from build123d import *

# Parameters (mm, degrees)
F1_DEPTH  = 3
F3_DEPTH  = 25
F4_R      = 5
F5_R      = 11.15
F5_R_2    = 2.65
F6_DEPTH  = 25
F7_W      = 78
F7_H      = 55.5
F7_R      = 2
F8_DEPTH  = 25
F9_R      = 8.15
F10_DEPTH = 25
F12_W     = 307.7535755343
F12_H     = 117.255145081
F13_DEPTH = 25
F14_W     = 20
F14_H     = 100
F15_DEPTH = 1.5
F17_DEPTH = 1.5
F19_DEPTH = 25


with BuildPart() as f1:
    # F0 (on Top) → F1 (new body)
    with BuildSketch(Plane.XY):
        with BuildLine():
            Line((-197.8147600734, 20.7911690818), (-202.2340594865, 0))
            Line((-202.2340594865, 0), (216.0975214603, 0))
            Line((216.0975214603, 0), (209.2885731253, 20.7911690818))
            ThreePointArc((209.2885731253, 20.7911690818), (167.4870934164, 78.1154778874), (100, 100))
            Line((100, 100), (-100, 100))
            ThreePointArc((-100, 100), (-162.932039105, 77.7145961457), (-197.8147600734, 20.7911690818))
        make_face()
    extrude(amount=F1_DEPTH)

    # F2 (on face) → F3 (cut)
    with BuildSketch(Plane.XY.offset(3)):
        with BuildLine():
            ThreePointArc((1.5842979518, 0), (9.4530988092, 4.1693984068), (12.6, 12.5))
            ThreePointArc((12.6, 12.5), (12.2192388124, 15.5741182224), (11.0999678023, 18.4624420155))
            ThreePointArc((11.0999678023, 18.4624420155), (0, 25.1), (-11.0999678023, 18.4624420155))
            ThreePointArc((-11.0999678023, 18.4624420155), (-11.1999147641, 6.7274867453), (-1.5842979518, 0))
            Line((-1.5842979518, 0), (1.5842979518, 0))
        make_face()
        with BuildLine():
            ThreePointArc((11.0999678023, 18.4624420155), (12.2192388124, 15.5741182224), (12.6, 12.5))
            ThreePointArc((12.6, 12.5), (9.4530988092, 4.1693984068), (1.5842979518, 0))
            Line((1.5842979518, 0), (21.7592636698, 0))
            Line((21.7592636698, 0), (11.0999678023, 18.4624420155))
        make_face()
        with BuildLine():
            ThreePointArc((-1.5842979518, 0), (0, -0.1), (1.5842979518, 0))
            Line((1.5842979518, 0), (-1.5842979518, 0))
        make_face()
        with BuildLine():
            ThreePointArc((-1.5842979518, 0), (-11.1999147641, 6.7274867453), (-11.0999678023, 18.4624420155))
            Line((-11.0999678023, 18.4624420155), (-21.7592636698, 0))
            Line((-21.7592636698, 0), (-1.5842979518, 0))
        make_face()
    extrude(amount=-F3_DEPTH, mode=Mode.SUBTRACT)

    # F4
    f4_edges = [f1.edges().sort_by_distance(p)[0] for p in [
        (-21.759264, 0, 1.5),
        (21.759264, 0, 1.5),
    ]]
    fillet(f4_edges, radius=F4_R)

    # F5 (on face) → F6 (cut)
    with BuildSketch(Plane.XY.offset(3)):
        Polygon((-145, 38.9489291724), (-152.75, 34.4744645862), (-152.75, 25.5255354138), (-145, 21.0510708276), (-137.25, 25.5255354138), (-137.25, 34.4744645862), align=None)
        with Locations((-115, 30)):
            Circle(F5_R)
        with Locations((-115, 60)):
            Circle(F5_R_2)
        with Locations((-145, 60)):
            Circle(F5_R_2)
    extrude(amount=-F6_DEPTH, mode=Mode.SUBTRACT)

    # F7 (on face) → F8 (cut)
    with BuildSketch(Plane.XY.offset(3)):
        with Locations((0, 57.75)):
            Rectangle(F7_W, F7_H)
        with Locations((-42.6313167033, 28.25)):
            Circle(F7_R)
        with Locations((-42.6313167033, 87.25)):
            Circle(F7_R)
        with Locations((42.3686832967, 87.25)):
            Circle(F7_R)
        with Locations((42.3686832967, 28.25)):
            Circle(F7_R)
    extrude(amount=-F8_DEPTH, mode=Mode.SUBTRACT)

    # F9 (on face) → F10 (cut)
    with BuildSketch(Plane.XY.offset(3)):
        with Locations((145, 30)):
            Circle(F9_R)
    extrude(amount=-F10_DEPTH, mode=Mode.SUBTRACT)

    # F12 (on face) → F13 (cut)
    with BuildSketch(Plane.XY.offset(3)):
        with Locations((-78.8767877671, 58.6275725405)):
            Rectangle(F12_W, F12_H)
    extrude(amount=-F13_DEPTH, mode=Mode.SUBTRACT)

    # F14 (on face) → F15 (cut)
    with BuildSketch(Plane(origin=(0, 0, 0), x_dir=(1, 0, 0), z_dir=(0, 0, -1))):
        with Locations((85, -50)):
            Rectangle(F14_W, F14_H)
    extrude(amount=-F15_DEPTH, mode=Mode.SUBTRACT)

    # F16 (on face) → F17 (join)
    with BuildSketch(Plane.XY.offset(3)):
        Polygon((75, 0), (75, 100), (62.6, 100), (69.6, 0), align=None)
    extrude(amount=-F17_DEPTH)

    # F18 (on face) → F19 (cut)
    with BuildSketch(Plane.XY.offset(3)):
        with BuildLine():
            ThreePointArc((198.5084757314, 61.1607791283), (200.0253825343, 64.4319411082), (200.5454428122, 68))
            ThreePointArc((200.5454428122, 68), (182.1177116525, 79.0050898814), (181.1675222846, 57.562365727))
            ThreePointArc((181.1675222846, 57.562365727), (182.9183296915, 56.599881095), (184.8001189484, 55.9286341693))
            ThreePointArc((184.8001189484, 55.9286341693), (188.4244577932, 67.0069708263), (198.5084757314, 61.1607791283))
        make_face()
        with BuildLine():
            ThreePointArc((184.8001189484, 55.9286341693), (182.9183296915, 56.599881095), (181.1675222846, 57.562365727))
            Line((181.1675222846, 57.562365727), (186.9720950966, 53.7374194362))
            ThreePointArc((186.9720950966, 53.7374194362), (185.772214529, 54.7201342708), (184.8001189484, 55.9286341693))
        make_face()
        with BuildLine():
            ThreePointArc((198.5988474131, 60), (198.5762203605, 60.5821458635), (198.5084757314, 61.1607791283))
            ThreePointArc((198.5084757314, 61.1607791283), (192.5027588454, 56.3217152895), (184.8001189484, 55.9286341693))
            ThreePointArc((184.8001189484, 55.9286341693), (185.772214529, 54.7201342708), (186.9720950966, 53.7374194362))
            ThreePointArc((186.9720950966, 53.7374194362), (194.655486109, 53.3969460712), (198.5988474131, 60))
        make_face()
        with BuildLine():
            ThreePointArc((184.8001189484, 55.9286341693), (192.5027588454, 56.3217152895), (198.5084757314, 61.1607791283))
            ThreePointArc((198.5084757314, 61.1607791283), (188.4244577932, 67.0069708263), (184.8001189484, 55.9286341693))
        make_face()
    extrude(amount=-F19_DEPTH, mode=Mode.SUBTRACT)


solid = f1.part
Geometry: final body of the model. Coordinates: model frame, mm. A direction names the side the tool comes from. Coordinates: 2 decimals unless noted, no trailing zeros. Order: outer loops, then holes, each group sorted by start corner. A loop starts at its lowest first (then second) coordinate and runs counter-clockwise, first axis right, second up. Notation, with made-up numbers: (71.25, 61) - (96.25, 61) arc R31 ccw to (96.25, 90) - close; hole circle Ø7 at (26, 40). An arc over 180 degrees is marked (long way). Use one line per item in the form item = value.
1) Section C-C (x = 79.5). Return loops of the section in (y, z).
Solutions:
outline = (0, 1.5) - (100, 1.5) - (100, 3) - (0, 3) - close
2) Section B-B (x = 145). Return loops of the section in (y, z).
Solutions:
outline = (0, 0) - (21.85, 0) - (21.85, 3) - (0, 3) - close; (38.15, 0) - (90.83, 0) - (90.83, 3) - (38.15, 3) - close
3) Set-up query: faces 4 (the face through (212.74, 10.25, 1.48)), 5 (the face through (79, 51, 1.5)). Return all of +Z, -Z, +X, -X, +Y, -Y with unobstructed straight access to the full face (end or side cutting, diameter ignored); none if empty.
Solutions:
face_4 = +Z, -Z, +X, +Y
face_5 = -Z, -X, +Y, -Y
4) Mould query, pull axis Y, two halves, no side actions, for faces 1 (the face through (66.05, 50.7, 2.26)), 2 (the face through (136.858, 30.358, 1.521)), 3 (the face through (184.029, 55.677, 1.521)). Classes: +Y half, -Y half, draft (parallel to the pull), parting line (faces both ways), or undercut.
Solutions:
face_1 = -Y half
face_2 = undercut
face_3 = +Y half
5) Pin query (flat end, axial travel): pin 1 (1.2 mm diameter, centred on y = 45, z = 1, fed in from -X); pin 2 (1.5 mm diameter, centred on y = 21, z = 1.5, fed in from +X). Return the tip coordinate at first contact, or that it passes through.
Solutions:
pin_1 = 66.43
pin_2 = 209.47
6) Ray query, L1, parallel to Y at x = 145, z = 0.7; L2, parallel to X at y = 31, z = 0.6; L3, parallel to Y at x = 146, z = 1.9. Return the intervals inside material, ascending.
Solutions:
L1 = 0 to 21.85, 38.15 to 90.83
L2 = 95 to 136.91, 153.09 to 205.4
L3 = 0 to 21.91, 38.09 to 90.4
7) Section A-A (y = 30). Return loops of the section in (x, z).
Solutions:
outline = (67.5, 1.5) - (95, 1.5) - (95, 0) - (136.85, 0) - (136.85, 3) - (67.5, 3) - close; (153.15, 0) - (205.83, 0) - (205.83, 3) - (153.15, 3) - close
8) Section D-D (y = 79.5). Return loops of the section in (x, z) (3 decimals).
Solutions:
outline = (64.035, 1.5) - (95, 1.5) - (95, 0) - (165.534, 0) - (165.534, 3) - (64.035, 3) - close
